```python
from build123d import *

# Parameters (mm, degrees)
F0_W     = 101.6
F0_H     = 101.6
F0_W_2   = 100.9904
F0_H_2   = 100.9904
F1_DEPTH = 254
F2_DEPTH = 254
F3_W     = 50.8
F3_H     = 58.6486
F4_DEPTH = 0.32766


with BuildPart() as f1:
    # F0 (on Top) → F1 (new body, symmetric)
    with BuildSketch(Plane.XY):
        Rectangle(F0_W, F0_H)
        Rectangle(F0_W_2, F0_H_2, mode=Mode.SUBTRACT)
    extrude(amount=F1_DEPTH, both=True)

    # F0 (on Top) → F2 (cut, symmetric)
    with BuildSketch(Plane.XY):
        Rectangle(F0_W_2, F0_H_2)
    extrude(amount=F2_DEPTH, both=True, mode=Mode.SUBTRACT)

    # F3 (on face) → F4 (cut)
    with BuildSketch(Plane.XZ.offset(50.8)):
        with Locations((0, -148.4757)):
            Rectangle(F3_W, F3_H)
    extrude(amount=-F4_DEPTH, mode=Mode.SUBTRACT)


solid = f1.part
```
Here's how the part is built. I have some questions about the finished solid (model axes, mm). A direction names the side the tool comes from. Coordinates: 2 decimals unless noted, no trailing zeros. Write each loop counter-clockwise with the first axis right and the second up, starting at its lowest first coordinate (ties: lowest second). Pieces come first, ordered by that corner, then holes. Notation, with made-up numbers: M 68.5,2 L 119.5,2 A13 ccw 119.5,11 Z; hole C -35.75,78 d10. An arc over 180 degrees is marked long. Answer as CSV lines item,"result". Start each with the question number.
Q1. I need wall thicknesses on probe 1 along X at (y, z) = (9.5, -44.5). Which ranges of the line are inside material? Lowest first, please. Write a range as [from, to].
Q2. For faces 4 (the flat face through (-50.8, -1, 4)), 5 (the flat face through (-1, 50.495, 4)), which set-ups out of +Z, -Z, +X, -X, +Y, -Y let a thin tool reach every point of the face, with its end or its side?
Q3. If we mould it in two halves opening along X, with no side actions, what happens to faces 1 (the flat face through (50.495, -1, 4)), 2 (the flat face through (50.8, -1, 4)), 3 (the flat face through (-1, 50.8, 4))? For each: pulls with the +X half, pulls with the -X half, needs draft (parallel to the pull), parting line crosses it, or undercut.
Q4. Suppose I cut it at B-B, the plane y = -37.5. List the corners of the cut face in (x, z) for me.
Q5. Suppose I cut it at A-A, the plane x = -6. List the corners of the cut face in (y, z) for me.
Q6. Suppose I cut it at D-D, the plane z = -86.5. List the corners of the cut face in (x, y) for me, then the cut area to 3 significant figures.
Entries:
1,probe 1,"x = [-50.8, -50.5], [50.5, 50.8]"
2,face 4,"+Z, -Z, -X, +Y, -Y"
2,face 5,"+Z, -Z"
3,face 1,"undercut"
3,face 2,"pulls with the +X half"
3,face 3,"needs draft"
4,outline,"M -50.8,-254 L -50.5,-254 L -50.5,254 L -50.8,254 Z; M 50.5,-254 L 50.8,-254 L 50.8,254 L 50.5,254 Z"
5,outline,"M -50.8,-254 L -50.5,-254 L -50.5,-177.8 L -50.8,-177.8 Z; M -50.8,-119.15 L -50.5,-119.15 L -50.5,254 L -50.8,254 Z; M 50.5,-254 L 50.8,-254 L 50.8,254 L 50.5,254 Z"
6,outline,"M -50.8,-50.8 L 50.8,-50.8 L 50.8,50.8 L -50.8,50.8 Z; hole M -50.5,-50.5 L 50.5,-50.5 L 50.5,50.5 L -50.5,50.5 Z"
6,area,"123 mm²"
